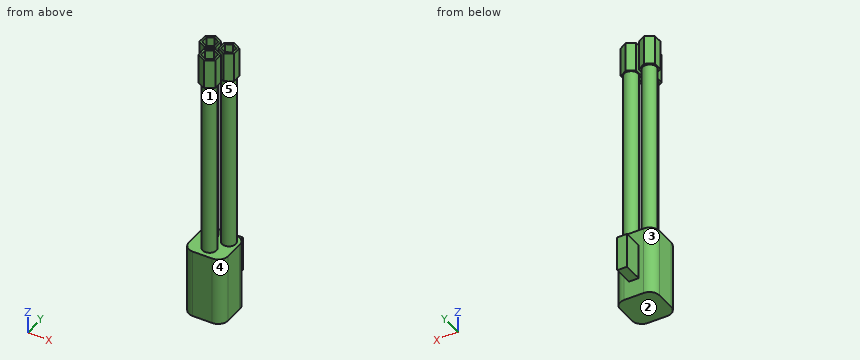
from build123d import *

# Parameters (mm, degrees)
IZIM1_W                          = 4
IZIM1_H                          = 4
Y_KSEKLIK_EKSTR_ZYON1_DEPTH      = 7
RADYUS1_R                        = 1
RADYUS2_R                        = 1
RADYUS3_R                        = 1
RADYUS4_R                        = 1
IZIM3_R                          = 0.7
IZIM3_R_2                        = 0.5
EKSTR_ZYON_NCE1_DEPTH            = 18
IZIM6_W                          = 3.561558411
IZIM6_H                          = 1.988004136
Y_KSEKLIK_EKSTR_ZYON2_DEPTH      = 0.5
Y_KSEKLIK_EKSTR_ZYON2_DEPTH_BACK = 0.5
EKSTR_ZYON_NCE3_DEPTH            = 3


with BuildPart() as part:
    # Çizim1 → Yükseklik-Ekstrüzyon1 (new body)
    with BuildSketch(Plane.XY):
        with Locations((0, -0.353018955)):
            Rectangle(IZIM1_W, IZIM1_H)
    extrude(amount=Y_KSEKLIK_EKSTR_ZYON1_DEPTH)

    # Radyus1
    radyus1_edges = [part.edges().sort_by_distance(p)[0] for p in [
        (2, -2.353018955, 3.5),
    ]]
    fillet(radyus1_edges, radius=RADYUS1_R)

    # Radyus2
    radyus2_edges = [part.edges().sort_by_distance(p)[0] for p in [
        (-2, 1.646981045, 3.5),
    ]]
    fillet(radyus2_edges, radius=RADYUS2_R)

    # Radyus3
    radyus3_edges = [part.edges().sort_by_distance(p)[0] for p in [
        (2, 1.646981045, 3.5),
    ]]
    fillet(radyus3_edges, radius=RADYUS3_R)

    # Radyus4
    radyus4_edges = [part.edges().sort_by_distance(p)[0] for p in [
        (-2, -2.353018955, 3.5),
    ]]
    fillet(radyus4_edges, radius=RADYUS4_R)

    # Çizim3 → Ekstrüzyon-İnce1 (add)
    with BuildSketch(Plane.XY.offset(7)):
        with Locations((-0.949214627, 0.542466542)):
            Circle(IZIM3_R)
        with Locations((-0.949214627, 0.542466542)):
            Circle(IZIM3_R_2, mode=Mode.SUBTRACT)
        with Locations((0.949214627, 0.542466542)):
            Circle(IZIM3_R)
        with Locations((0.949214627, 0.542466542)):
            Circle(IZIM3_R_2, mode=Mode.SUBTRACT)
        with Locations((0, -1.147016096)):
            Circle(IZIM3_R)
        with Locations((0, -1.147016096)):
            Circle(IZIM3_R_2, mode=Mode.SUBTRACT)
    extrude(amount=EKSTR_ZYON_NCE1_DEPTH)

    # Çizim6 → Yükseklik-Ekstrüzyon2 (add, two sides)
    with BuildSketch(Plane(origin=(0, 0, 0), x_dir=(0, 0, -1), z_dir=(1, 0, 0))) as y_kseklik_ekstr_zyon2_sk:
        with Locations((-3.576903913, 2.640983113)):
            Rectangle(IZIM6_W, IZIM6_H)
    extrude(amount=Y_KSEKLIK_EKSTR_ZYON2_DEPTH)
    extrude(y_kseklik_ekstr_zyon2_sk.sketch, amount=-Y_KSEKLIK_EKSTR_ZYON2_DEPTH_BACK)

    # Çizim4 → Ekstrüzyon-İnce3 (add)
    with BuildSketch(Plane.XY.offset(25)):
        Polygon((-0.949214627, -0.409912915), (-0.124429823, 0.066276814), (-0.124429823, 1.018656271), (-0.949214627, 1.494845999), (-1.773999431, 1.018656271), (-1.773999431, 0.066276814), align=None)
        Polygon((-0.949214627, -0.178972807), (-0.324429823, 0.181746867), (-0.324429823, 0.903186217), (-0.949214627, 1.263905891), (-1.573999431, 0.903186217), (-1.573999431, 0.181746867), align=None, mode=Mode.SUBTRACT)
        Polygon((0.949214627, -0.371158962), (1.740437522, 0.08565379), (1.740437522, 0.999279294), (0.949214627, 1.456092046), (0.157991731, 0.999279294), (0.157991731, 0.08565379), align=None)
        Polygon((0.949214627, -0.140218854), (1.540437522, 0.201123844), (1.540437522, 0.88380924), (0.949214627, 1.225151938), (0.357991731, 0.88380924), (0.357991731, 0.201123844), align=None, mode=Mode.SUBTRACT)
        Polygon((0.871605884, -1.606698651), (0.833899712, -0.622024536), (-0.037706171, -0.162341981), (-0.871605884, -0.687333541), (-0.833899712, -1.672007655), (0.037706171, -2.131690211), align=None)
        Polygon((0.667333897, -1.498966164), (0.638464649, -0.745063023), (-0.028869248, -0.393112954), (-0.667333897, -0.795066027), (-0.638464649, -1.548969169), (0.028869248, -1.900919237), align=None, mode=Mode.SUBTRACT)
    extrude(amount=EKSTR_ZYON_NCE3_DEPTH)


solid = part.part
Could you check a few things on this model? Use its own coordinates, in mm. Face numbers are marked on the shaded views. A direction names the side the tool comes from. Round coordinates to 2 decimals unless told otherwise and drop trailing zeros. Loops run counter-clockwise (first coordinate to the right, second up) from the corner with the lowest first, then second, coordinate; pieces in that order, holes last. Notation, with made-up numbers: (-11, 89.25) -> (31, 89.25) arc R16 ccw to (31, 108.25) -> close; hole circle Ø9 at (87.5, 11). An arc over 180 degrees is marked (long way). Use CSV: the item, a comma, the result in double quotes.
(1) If I drill on probe 1 along Z at (x, y) = (0.35, -1.9); probe 2 along Y at (x, z) = (0, 19); probe 3 along X at (y, z) = (2.5, 4.25), over which ranges is the centre line in solid material (lowest first)? Write a range as [from, to].
Return value:
probe 1,"z = [0, 7], [25, 28]"
probe 2,"y = [-1.85, -1.65], [-0.65, -0.45]"
probe 3,"x = [-0.5, 0.5]"
(2) If we mould it in two halves opening along Z, with no side actions, what happens to the marked faces 1, 2 and 3? For each: +Z half, -Z half, draft (parallel to the pull), parting line (faces both ways), or undercut.
Return value:
face 1,"undercut"
face 2,"-Z half"
face 3,"draft"
(3) Suppose I cut it at C-C on z = 14.25. Write out the boundary of the cut face in (x, y).
Return value:
outline,"circle Ø1.4 at (-0.95, 0.54); circle Ø1.4 at (0, -1.15); circle Ø1.4 at (0.95, 0.54); hole circle Ø1 at (-0.95, 0.54); hole circle Ø1 at (0, -1.15); hole circle Ø1 at (0.95, 0.54)"
(4) Suppose I cut it at A-A on z = 26. Give the number of separate pieces and of enclosed holes in the cut face, plus the area to 3 significant figures.
Return value:
separate pieces,"3"
enclosed holes,"3"
area,"3.01 mm²"
(5) For the marked faces 4 and 5, which set-ups out of +Z, -Z, +X, -X, +Y, -Y let a thin tool reach every point of the face, with its end or its side?
Return value:
face 4,"+Z, -Z, +X, -Y"
face 5,"none"
(6) Will these pins go through, and if not, where does the flat tip stop? pin 1 Ø1.1 at (x, y) = (0, 2.5) entering from -Z; pin 2 Ø1.5 at (x, y) = (1, -1.5) entering from -Z; pin 3 Ø0.8 at (y, z) = (0.5, 27) entering from -X; pin 4 Ø1.6 at (y, z) = (2.5, 4) entering from -X.
Return value:
pin 1,"stops at z = 1.8"
pin 2,"stops at z = 0"
pin 3,"stops at x = -1.77"
pin 4,"stops at x = -0.5"
(7) Suppose I cut it at B-B on y = 2. Write out the boundary of the cut face in (x, z).
Return value:
outline,"(-0.5, 1.8) -> (0.5, 1.8) -> (0.5, 5.36) -> (-0.5, 5.36) -> close"
